The model under review builds one solid part; all positions refer to its coordinate system, in mm. A direction names the side the tool comes from. Coordinates: 2 decimals unless noted, no trailing zeros. Write each loop counter-clockwise with the first axis right and the second up, starting at its lowest first coordinate (ties: lowest second). Pieces come first, ordered by that corner, then holes. Notation, with made-up numbers: (39.25, 26) - (96.25, 26) arc R18 ccw to (96.25, 50) - close; hole circle Ø1 at (50.5, 82). An arc over 180 degrees is marked (long way). Use one line per item in the form item = value. Start each with the question number.
```python
from build123d import *

# Parameters (mm, degrees)
CYLINDER002_R     = 11.1
CYLINDER002_DEPTH = 7
TORUS002_R        = 10
CYLINDER001_R     = 11.1
CYLINDER001_DEPTH = 7
CYLINDER_R        = 15
CYLINDER_DEPTH    = 20
CYLINDER003_R     = 19
CYLINDER003_DEPTH = 10


with BuildPart() as cylinder002:
    # Cylinder002 → Cylinder002 (new body)
    with BuildSketch(Plane.XY.offset(13)):
        Circle(CYLINDER002_R)
    extrude(amount=CYLINDER002_DEPTH)


with BuildPart() as cone:
    # Cone → Cone (revolve)
    with BuildSketch(Plane(origin=(0, 0, 7), x_dir=(1, 0, 0), z_dir=(0, -1, 0))):
        Polygon((0, 0), (11, 0), (0, 11), align=None)
    revolve(axis=Axis((0, 0, 7), (0, 0, 1)))


with BuildPart() as cone001:
    # Cone001 → Cone001 (revolve)
    with BuildSketch(Plane(origin=(0, 0, 13), x_dir=(-1, 0, 0), z_dir=(0, -1, 0))):
        Polygon((0, 0), (11, 0), (0, 11), align=None)
    revolve(axis=Axis((0, 0, 13), (0, 0, -1)))


with BuildPart() as torus002:
    # Torus002 → Torus002 (revolve)
    with BuildSketch(Plane(origin=(0, 0, 10), x_dir=(1, 0, 0), z_dir=(0, -1, 0))):
        with Locations((25, 0)):
            Circle(TORUS002_R)
    revolve(axis=Axis((0, 0, 10), (0, 0, 1)))


with BuildPart() as negativefusion:
    # Cylinder001 → Cylinder001 (new body)
    with BuildSketch(Plane.XY):
        Circle(CYLINDER001_R)
    extrude(amount=CYLINDER001_DEPTH)

    # Fusion: union Cylinder002, Cone, Cone001, Torus002
    add(cylinder002.part)
    add(cone.part)
    add(cone001.part)
    add(torus002.part)


with BuildPart() as cylinder:
    # Cylinder → Cylinder (new body)
    with BuildSketch(Plane.XY):
        Circle(CYLINDER_R)
    extrude(amount=CYLINDER_DEPTH)


with BuildPart() as cut:
    # Cylinder003 → Cylinder003 (new body)
    with BuildSketch(Plane.XY):
        Circle(CYLINDER003_R)
    extrude(amount=CYLINDER003_DEPTH)

    # Fusion001: union Cylinder
    add(cylinder.part)

    # Cut: cut NegativeFusion
    add(negativefusion.part, mode=Mode.SUBTRACT)


solid = cut.part
```
1. Take a section at C-C (z = 17). State the section outline as (x, y) points, plus the area to 3 significant figures.
2. The part is to be moulded in two halves that separate along X. For faces 1 (the flat face through (2.2, 11.2, 20)), 2 (the cylindrical face through (-14.985, 0.66, 14.93)), 3 (the conical face through (-7.77, 2.447, 10.146)), say which applies: released by +X, released by -X, zero draft, split by the parting line, or undercut.
3. Take a section at A-A (y = 0). State the section outline as (x, z) points, plus the area to 3 significant figures.
4. For L1, parallel to Y at x = 0, z = 17.5; L2, parallel to Y at x = 8, z = 15.25; L3, parallel to X at y = -3, z = 17.75, list the stretches that pass through material, from the lowest coordinate up.
5. For P1, Ø6.5, axis at x = 2.5, y = -3, coming from the -Z side; P2, Ø2, axis at x = -11, y = 0.5, coming from the +Z side; P3, Ø4, axis at y = 1.5, z = 5, coming from the +X side; P4, Ø2, axis at y = 12.5, z = 12.5, coming from the -X side, all flat-tipped, find the tip position at first contact; note any pin that passes through.
6. Take a section at D-D (z = 4.5). State the section outline as (x, y) points.
7. For faces 4 (the cylindrical face through (5.97, 9.36, 3.45)), 5 (the cylindrical face through (8.767, -16.856, 0.986)), 6 (the cylindrical face through (5.97, 9.36, 16.45)), list the 3-axis set-ups (+Z, -Z, +X, -X, +Y, -Y) from which the entire face can be reached by the end or side of a thin tool; tool diameter is ignored.
Returned:
q1.outline = circle Ø30 at (0, 0); hole circle Ø22.2 at (0, 0)
q1.area = 320 mm²
q2.face_1 = zero draft
q2.face_2 = split by the parting line
q2.face_3 = undercut
q3.outline = (-19, 0) - (-11.1, 0) - (-11.1, 7) - (-11, 7) - (-8, 10) - (-11, 13) - (-11.1, 13) - (-11.1, 20) - (-15, 20) - (-15, 10) arc R10 cw to (-19, 2) - close; (8, 10) - (11, 7) - (11.1, 7) - (11.1, 0) - (19, 0) - (19, 2) arc R10 cw to (15, 10) - (15, 20) - (11.1, 20) - (11.1, 13) - (11, 13) - close
q3.area = 210 mm²
q4.L1 = -15 to -11.1, 11.1 to 15
q4.L2 = -12.69 to -7.69, 7.69 to 12.69
q4.L3 = -14.7 to -10.69, 10.69 to 14.7
q5.P1 = through
q5.P2 = 20
q5.P3 = 17.8
q5.P4 = -9.63
q6.outline = circle Ø33.3 at (0, 0); hole circle Ø22.2 at (0, 0)
q7.face_4 = -Z
q7.face_5 = +Z, -Z
q7.face_6 = +Z
